Can you work these out from the model? Positions are in its coordinate system, mm. Face numbers are marked on the shaded views. Coordinates: 2 decimals unless noted, no trailing zeros. Order: outer loops, then holes, each group sorted by start corner. A loop starts at its lowest first (then second) coordinate and runs counter-clockwise, first axis right, second up.
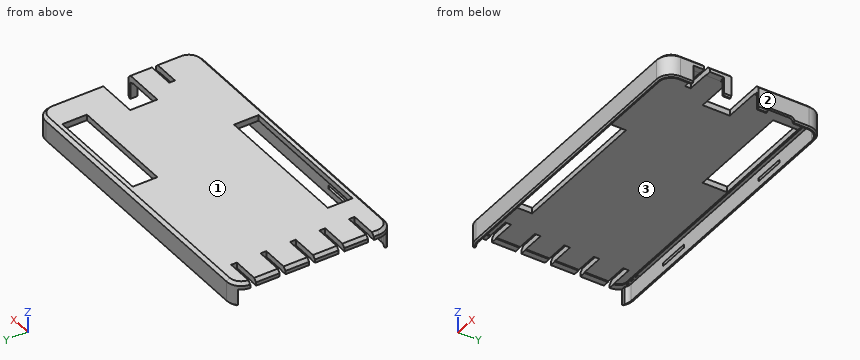
```python
from build123d import *

# Parameters (mm, degrees)
PAD006_DEPTH               = 8.3
POCKET_DEPTH               = 6
PAD006_MIRRORED010_2_DEPTH = 8.3
POCKET_MIRRORED010_2_DEPTH = 6
PAD007_DEPTH               = 2
PAD007_MIRRORED014_2_DEPTH = 2
POCKET003_DEPTH            = 30.5
PAD009_DEPTH               = 19.5
PAD009_FACE36_W            = 39
PAD009_FACE36_H            = 1.2
POCKET004_DEPTH            = 0.2
CHAMFER005_SIZE            = 0.5
CHAMFER006_SIZE            = 1
CHAMFER007_SIZE            = 0.2999
SKETCH030_W                = 49
SKETCH030_H                = 8.5
SKETCH030_W_2              = 36.8
POCKET010_DEPTH            = 5
POCKET011_DEPTH            = 10
SKETCH018_W                = 9.4
SKETCH018_H                = 50
POCKET012_DEPTH            = 15
POCKET013_DEPTH            = 5
POCKET014_DEPTH            = 10
POCKET015_DEPTH            = 10
POCKET016_DEPTH            = 10
POCKET017_DEPTH            = 10
POCKET018_DEPTH            = 10


with BuildPart() as part:
    # Sketch008 (on DatumPlane) → Pad006 (new body)
    with BuildSketch(Plane.XY.offset(17.8)):
        with BuildLine():
            ThreePointArc((-47.2, 27.2), (-50.735534, 25.735534), (-52.2, 22.2))
            Line((-52.2, 0), (-52.2, 22.2))
            Line((-50.2, 0), (-52.2, 0))
            Line((-50.2, 22.2), (-50.2, 0))
            ThreePointArc((-47.2, 25.2), (-49.32132, 24.32132), (-50.2, 22.2))
            Line((0, 25.2), (-47.2, 25.2))
            Line((0, 27.2), (0, 25.2))
            Line((-47.2, 27.2), (0, 27.2))
        make_face()
    pad006 = extrude(amount=-PAD006_DEPTH)

    # Sketch009 (on Face10 of Pad006) → Pocket (cut)
    with BuildSketch(Plane(origin=(0, 0, 9.5), x_dir=(1, 0, 0), z_dir=(0, 0, -1))):
        with BuildLine():
            ThreePointArc((-50.2, -22.2), (-49.32132, -24.32132), (-47.2, -25.2))
            Line((-47.2, -25.2), (0, -25.2))
            Line((0, -25.2), (0, -26.3))
            Line((0, -26.3), (-47.2, -26.3))
            ThreePointArc((-51.3, -22.2), (-50.099138, -25.099138), (-47.2, -26.3))
            Line((-51.3, 0), (-51.3, -22.2))
            Line((-50.2, 0), (-51.3, 0))
            Line((-50.2, -22.2), (-50.2, 0))
        make_face()
    pocket = extrude(amount=-POCKET_DEPTH, mode=Mode.SUBTRACT)

    # Sketch008 Mirrored010 2 → Pad006 Mirrored010 2 (add)
    with BuildSketch(Plane(origin=(0, 0, 17.8), x_dir=(-1, 0, 0), z_dir=(0, 0, -1))):
        with BuildLine():
            ThreePointArc((-47.2, 27.2), (-50.735534, 25.735534), (-52.2, 22.2))
            Line((-52.2, 0), (-52.2, 22.2))
            Line((-50.2, 0), (-52.2, 0))
            Line((-50.2, 22.2), (-50.2, 0))
            ThreePointArc((-47.2, 25.2), (-49.32132, 24.32132), (-50.2, 22.2))
            Line((0, 25.2), (-47.2, 25.2))
            Line((0, 27.2), (0, 25.2))
            Line((-47.2, 27.2), (0, 27.2))
        make_face()
    pad006_mirrored010_2 = extrude(amount=PAD006_MIRRORED010_2_DEPTH)

    # Sketch009 Mirrored010 2 → Pocket Mirrored010 2 (cut)
    with BuildSketch(Plane(origin=(0, 0, 9.5), x_dir=(-1, 0, 0), z_dir=(0, 0, 1))):
        with BuildLine():
            ThreePointArc((-50.2, -22.2), (-49.32132, -24.32132), (-47.2, -25.2))
            Line((-47.2, -25.2), (0, -25.2))
            Line((0, -25.2), (0, -26.3))
            Line((0, -26.3), (-47.2, -26.3))
            ThreePointArc((-51.3, -22.2), (-50.099138, -25.099138), (-47.2, -26.3))
            Line((-51.3, 0), (-51.3, -22.2))
            Line((-50.2, 0), (-51.3, 0))
            Line((-50.2, -22.2), (-50.2, 0))
        make_face()
    pocket_mirrored010_2 = extrude(amount=POCKET_MIRRORED010_2_DEPTH, mode=Mode.SUBTRACT)

    # Mirrored011: Pad006, Pocket, Pad006 Mirrored010 2, Pocket Mirrored010 2 across Sketch008 H_Axis
    add(pad006.mirror(Plane(origin=(0, 0, 17.8), x_dir=(0, 0, 1), z_dir=(0, 1, 0))))
    add(pocket.mirror(Plane(origin=(0, 0, 17.8), x_dir=(0, 0, 1), z_dir=(0, 1, 0))), mode=Mode.SUBTRACT)
    add(pad006_mirrored010_2.mirror(Plane(origin=(0, 0, 17.8), x_dir=(0, 0, 1), z_dir=(0, 1, 0))))
    add(pocket_mirrored010_2.mirror(Plane(origin=(0, 0, 17.8), x_dir=(0, 0, 1), z_dir=(0, 1, 0))), mode=Mode.SUBTRACT)

    # Sketch011 (on DatumPlane) → Pad007 (join)
    with BuildSketch(Plane.XY.offset(17.8)):
        with BuildLine():
            ThreePointArc((-47.2, 25.2), (-49.32132, 24.32132), (-50.2, 22.2))
            Line((-50.2, 22.2), (-50.2, 0))
            Line((-50.2, 0), (0, 0))
            Line((0, 0), (0, 25.2))
            Line((0, 25.2), (-47.2, 25.2))
        make_face()
    pad007 = extrude(amount=-PAD007_DEPTH)

    # Sketch011 Mirrored014 2 → Pad007 Mirrored014 2 (add)
    with BuildSketch(Plane(origin=(0, 0, 17.8), x_dir=(-1, 0, 0), z_dir=(0, 0, -1))):
        with BuildLine():
            ThreePointArc((-47.2, 25.2), (-49.32132, 24.32132), (-50.2, 22.2))
            Line((-50.2, 22.2), (-50.2, 0))
            Line((-50.2, 0), (0, 0))
            Line((0, 0), (0, 25.2))
            Line((0, 25.2), (-47.2, 25.2))
        make_face()
    pad007_mirrored014_2 = extrude(amount=PAD007_MIRRORED014_2_DEPTH)

    # Mirrored015: Pad007, Pad007 Mirrored014 2 across Sketch011 H_Axis
    add(pad007.mirror(Plane(origin=(0, 0, 17.8), x_dir=(0, 0, 1), z_dir=(0, 1, 0))))
    add(pad007_mirrored014_2.mirror(Plane(origin=(0, 0, 17.8), x_dir=(0, 0, 1), z_dir=(0, 1, 0))))

    # Sketch013 → Pocket003 (cut, symmetric)
    with BuildSketch(Plane.YZ):
        with BuildLine():
            ThreePointArc((-26.1, 12.9), (-26.7, 12.3), (-26.1, 11.7))
            Line((-26.1, 12.9), (-26.1, 11.7))
        make_face()
    pocket003 = extrude(amount=POCKET003_DEPTH, both=True, mode=Mode.SUBTRACT)

    # Sketch013 → Pad009 (join, symmetric)
    with BuildSketch(Plane.YZ):
        with BuildLine():
            ThreePointArc((-26.1, 12.9), (-26.7, 12.3), (-26.1, 11.7))
            Line((-26.1, 12.9), (-26.1, 11.7))
        make_face()
    pad009 = extrude(amount=PAD009_DEPTH, both=True)

    # Pad009 Face36 → Pocket004 (cut)
    with BuildSketch(Plane(origin=(0, -26.1, 12.3), x_dir=(1, 0, 0), z_dir=(0, 1, 0))):
        Rectangle(PAD009_FACE36_W, PAD009_FACE36_H)
    pocket004 = extrude(amount=-POCKET004_DEPTH, mode=Mode.SUBTRACT)

    # Mirrored017: Pocket003, Pad009, Pocket004 across Sketch013 V_Axis
    add(pocket003.mirror(Plane(origin=(0, 0, 0), x_dir=(1, 0, 0), z_dir=(0, 1, 0))), mode=Mode.SUBTRACT)
    add(pad009.mirror(Plane(origin=(0, 0, 0), x_dir=(1, 0, 0), z_dir=(0, 1, 0))))
    add(pocket004.mirror(Plane(origin=(0, 0, 0), x_dir=(1, 0, 0), z_dir=(0, 1, 0))), mode=Mode.SUBTRACT)

    # Chamfer005
    chamfer005_edges = [part.edges().sort_by_distance(p)[0] for p in [
        (0, -27.2, 9.5),
    ]]
    chamfer(chamfer005_edges, length=CHAMFER005_SIZE)

    # Chamfer006
    chamfer006_edges = [part.edges().sort_by_distance(p)[0] for p in [
        (0, -27.2, 17.8),
    ]]
    chamfer(chamfer006_edges, length=CHAMFER006_SIZE)

    # Chamfer007
    chamfer007_edges = [part.edges().sort_by_distance(p)[0] for p in [
        (50.2, 0, 15.8),
    ]]
    chamfer(chamfer007_edges, length=CHAMFER007_SIZE)

    # Sketch030 (on DatumPlane) → Pocket010 (cut)
    with BuildSketch(Plane.XY.offset(17.8)):
        with Locations((-9.76, -20.57)):
            Rectangle(SKETCH030_W, SKETCH030_H)
        with Locations((23.81, 20.57)):
            Rectangle(SKETCH030_W_2, SKETCH030_H)
    extrude(amount=-POCKET010_DEPTH, mode=Mode.SUBTRACT)

    # Sketch017 (on DatumPlane) → Pocket011 (cut)
    with BuildSketch(Plane.YZ.offset(52.2)):
        Polygon((-7.2, 7.6), (-7.2, 15.6), (-12.1, 15.6), (-12.1, 18.1), (-14.1, 18.1), (-14.1, 15.6), (-17.8, 15.6), (-17.8, 7.6), (-17.8, 2.6), (-7.2, 2.6), align=None)
    extrude(amount=-POCKET011_DEPTH, mode=Mode.SUBTRACT)

    # Sketch018 (on DatumPlane) → Pocket012 (cut)
    with BuildSketch(Plane.YZ.offset(52.2)):
        with Locations((0, -6)):
            Rectangle(SKETCH018_W, SKETCH018_H)
    extrude(amount=-POCKET012_DEPTH, mode=Mode.SUBTRACT)

    # Sketch019 (on DatumPlane) → Pocket013 (cut)
    with BuildSketch(Plane.YZ.offset(52.2)):
        with BuildLine():
            Line((7.9, -40.25), (7.9, 9.75))
            ThreePointArc((9.15, 11), (8.266117, 10.633883), (7.9, 9.75))
            Line((9.15, 11), (15.85, 11))
            ThreePointArc((17.1, 9.75), (16.733883, 10.633883), (15.85, 11))
            Line((17.1, 9.75), (17.1, -40.25))
            Line((7.9, -40.25), (17.1, -40.25))
        make_face()
    extrude(amount=-POCKET013_DEPTH, mode=Mode.SUBTRACT)

    # Sketch026 (on DatumPlane) → Pocket014 (cut)
    with BuildSketch(Plane(origin=(-52.2, 0, 0), x_dir=(0, -1, 0), z_dir=(-1, 0, 0))):
        Polygon((-15.02, 7.6), (-15.02, 15.6), (-20.32, 15.6), (-20.32, 18.1), (-22.32, 18.1), (-22.32, 15.6), (-25.62, 15.6), (-25.62, 7.6), (-25.62, -42.4), (-15.02, -42.4), align=None)
    extrude(amount=-POCKET014_DEPTH, mode=Mode.SUBTRACT)

    # Sketch027 (on DatumPlane) → Pocket015 (cut)
    with BuildSketch(Plane(origin=(-52.2, 0, 0), x_dir=(0, -1, 0), z_dir=(-1, 0, 0))):
        Polygon((-4.86, 7.6), (-4.86, 15.6), (-10.16, 15.6), (-10.16, 18.1), (-12.16, 18.1), (-12.16, 15.6), (-15.46, 15.6), (-15.46, 7.6), (-15.46, -42.4), (-4.86, -42.4), align=None)
    extrude(amount=-POCKET015_DEPTH, mode=Mode.SUBTRACT)

    # Sketch025 (on DatumPlane) → Pocket016 (cut)
    with BuildSketch(Plane(origin=(-52.2, 0, 0), x_dir=(0, -1, 0), z_dir=(-1, 0, 0))):
        Polygon((5.3, 7.6), (5.3, 15.6), (0, 15.6), (0, 18.1), (-2, 18.1), (-2, 15.6), (-5.3, 15.6), (-5.3, 7.6), (-5.3, -42.4), (5.3, -42.4), align=None)
    extrude(amount=-POCKET016_DEPTH, mode=Mode.SUBTRACT)

    # Sketch028 (on DatumPlane) → Pocket017 (cut)
    with BuildSketch(Plane(origin=(-52.2, 0, 0), x_dir=(0, -1, 0), z_dir=(-1, 0, 0))):
        Polygon((15.46, 7.6), (15.46, 15.6), (10.16, 15.6), (10.16, 18.1), (8.16, 18.1), (8.16, 15.6), (4.86, 15.6), (4.86, 7.6), (4.86, -42.4), (15.46, -42.4), align=None)
    extrude(amount=-POCKET017_DEPTH, mode=Mode.SUBTRACT)

    # Sketch029 (on DatumPlane) → Pocket018 (cut)
    with BuildSketch(Plane(origin=(-52.2, 0, 0), x_dir=(0, -1, 0), z_dir=(-1, 0, 0))):
        Polygon((25.62, 7.6), (25.62, 15.6), (20.32, 15.6), (20.32, 18.1), (18.32, 18.1), (18.32, 15.6), (15.02, 15.6), (15.02, 7.6), (15.02, -42.4), (25.62, -42.4), align=None)
    extrude(amount=-POCKET018_DEPTH, mode=Mode.SUBTRACT)


solid = part.part
```
1. Thinking about a two-plate mould opening in X: for the marked faces 1, 2 and 3, which applies, pulls with the +X half, pulls with the -X half, needs draft (parallel to the pull), parting line crosses it, or undercut?
Completed:
face 1: needs draft
face 2: pulls with the +X half
face 3: undercut
2. Please list where these lines run through material, in increasing order: probe 1 along Y at (x, z) = (20, 13); probe 2 along Y at (x, z) = (48, 16); probe 3 along Y at (x, z) = (-29, 16.75).
Completed:
probe 1: y = -27.2 to -26.3, 26.3 to 27.2
probe 2: y = -27.14 to -14.1, -12.1 to -4.7, 4.7 to 27.14
probe 3: y = -27.2 to -24.82, -16.32 to 27.2
3. I'm going to push flat-ended pins straight in: pin 1 (2.5 mm diameter, centred on x = -49, z = 16, fed in from -Y); pin 2 (6 mm diameter, centred on x = 12, y = -3.5, fed in from -Z); pin 3 (3 mm diameter, centred on y = -17, z = 12, fed in from -X); pin 4 (0.6 mm diameter, centred on y = -22.5, z = 17, fed in from +X). Where does each tip first touch, or does it pass through?
Completed:
pin 1: stops at y = -27.17
pin 2: stops at z = 15.8
pin 3: stops at x = 51.3
pin 4: stops at x = 52.2
4. Imagine slicing it at A-A on z = 14. Please give me the cut outline in (x, y), then the cut area to 3 significant figures.
Completed:
outline: (-50.85, -25.62) arc R5 ccw to (-47.2, -27.2) - (47.2, -27.2) arc R5 ccw to (52.2, -22.2) - (52.2, -17.8) - (51.3, -17.8) - (51.3, -22.2) arc R4.1 cw to (47.2, -26.3) - (-47.2, -26.3) arc R4.1 cw to (-49.46, -25.62) - close; (-50.85, 25.62) - (-49.46, 25.62) arc R4.1 cw to (-47.2, 26.3) - (47.2, 26.3) arc R4.1 cw to (51.3, 22.2) - (51.3, 4.7) - (52.2, 4.7) - (52.2, 22.2) arc R5 ccw to (47.2, 27.2) - (-47.2, 27.2) arc R5 ccw to start; (51.3, -7.2) - (52.2, -7.2) - (52.2, -4.7) - (51.3, -4.7) - close
area: 211 mm2
5. Imagine slicing it at D-D on x = 40. Give the number of separate pieces and of enclosed holes in the cut face, then the cut area to 3 significant figures.
Completed:
separate pieces: 3
enclosed holes: 0
area: 83.8 mm2
